```python
from build123d import *

# Parameters (mm, degrees)
PAD033_DEPTH            = 144
SKETCH060_R             = 1.5
POCKET025_DEPTH         = 7
POCKET026_DEPTH         = 4
SKETCH065_R             = 1.5
POCKET029_DEPTH         = 7
POCKET030_DEPTH         = 5
BODY018_ROLL_ANGLE      = 90
BODY018_PLACEMENT_ANGLE = 180


with BuildPart() as righthigh:
    # Sketch059 → Pad033 (new body)
    with BuildSketch(Plane.XZ):
        Polygon((0, 0), (0, 10), (-7, 10), (-7, 14), (4, 14), (4, 8), (7, 8), (7, -8), (4, -8), (4, -14), (-7, -14), (-7, -10), (0, -10), align=None)
    extrude(amount=PAD033_DEPTH)

    # Sketch060 (on Face6 of Pad033) → Pocket025 (cut)
    with BuildSketch(Plane(origin=(7, 0, 0), x_dir=(0, 0, 1), z_dir=(1, 0, 0))):
        with Locations((0, 120)):
            Circle(SKETCH060_R)
        with Locations((0, 20)):
            Circle(SKETCH060_R)
    extrude(amount=-POCKET025_DEPTH, mode=Mode.SUBTRACT)

    # Sketch061 (on Face12 of Pocket025) → Pocket026 (cut)
    with BuildSketch(Plane(origin=(7, 0, 0), x_dir=(0, 0, 1), z_dir=(1, 0, 0))):
        Polygon((3.176, 20), (1.588, 22.750497), (-1.588, 22.750497), (-3.176, 20), (-1.588, 17.249503), (1.588, 17.249503), align=None)
        Polygon((3.176, 120), (1.588, 122.750497), (-1.588, 122.750497), (-3.176, 120), (-1.588, 117.249503), (1.588, 117.249503), align=None)
    extrude(amount=-POCKET026_DEPTH, mode=Mode.SUBTRACT)

    # Sketch065 (on Face2 of Pocket026) → Pocket029 (cut)
    with BuildSketch(Plane(origin=(0, 0, 0), x_dir=(0, 0, -1), z_dir=(-1, 0, 0))):
        with Locations((0, 12.5)):
            Circle(SKETCH065_R)
        with Locations((0, 37.5)):
            Circle(SKETCH065_R)
        with Locations((0, 62.5)):
            Circle(SKETCH065_R)
        with Locations((0, 87.5)):
            Circle(SKETCH065_R)
        with Locations((0, 112.5)):
            Circle(SKETCH065_R)
        with Locations((0, 137.5)):
            Circle(SKETCH065_R)
    extrude(amount=-POCKET029_DEPTH, mode=Mode.SUBTRACT)

    # Sketch066 → Pocket030 (cut)
    with BuildSketch(Plane(origin=(0, 0, 0), x_dir=(0, 0, -1), z_dir=(-1, 0, 0))):
        Polygon((3.175366, 12.563434), (1.532748, 15.281665), (-1.642619, 15.218231), (-3.175366, 12.436566), (-1.532748, 9.718335), (1.642619, 9.781769), align=None)
        Polygon((3.175984, 37.50994), (1.579384, 40.255453), (-1.5966, 40.245513), (-3.175984, 37.49006), (-1.579384, 34.744547), (1.5966, 34.754487), align=None)
        Polygon((3.176, 62.500829), (1.587282, 65.250911), (-1.588718, 65.250082), (-3.176, 62.499171), (-1.587282, 59.749089), (1.588718, 59.749918), align=None)
        Polygon((3.176, 87.500019), (1.587984, 90.250506), (-1.588016, 90.250487), (-3.176, 87.499981), (-1.587984, 84.749494), (1.588016, 84.749513), align=None)
        Polygon((3.176, 112.5), (1.588, 115.250497), (-1.588, 115.250497), (-3.176, 112.5), (-1.588, 109.749503), (1.588, 109.749503), align=None)
        Polygon((3.176, 137.5), (1.588, 140.250497), (-1.588, 140.250497), (-3.176, 137.5), (-1.588, 134.749503), (1.588, 134.749503), align=None)
    extrude(amount=-POCKET030_DEPTH, mode=Mode.SUBTRACT)


with BuildPart() as righthigh_1:
    # Body018 roll: moved
    add(righthigh.part.rotate(Axis((0, 0, 0), (1, 0, 0)), BODY018_ROLL_ANGLE))


with BuildPart() as righthigh_2:
    # Body018 placement: moved
    add(righthigh_1.part.moved(Location((120, -275.5, 350))).rotate(Axis((120, -275.5, 350), (0, 0, 1)), BODY018_PLACEMENT_ANGLE))


with BuildPart() as lefthigh:
    # Part__Mirroring007: instance of RightHigh
    add(righthigh_2.part.mirror(Plane(origin=(0, 0, 0), x_dir=(0, -1, 0), z_dir=(1, 0, 0))))


solid = lefthigh.part
```
Model file for the job. Use its own axes, mm. A direction names the side the tool comes from. Coordinates: 2 decimals unless noted, no trailing zeros. Write each loop counter-clockwise with the first axis right and the second up, starting at its lowest first coordinate (ties: lowest second). Pieces come first, ordered by that corner, then holes. Notation, with made-up numbers: (-14, 47) - (0, 47) arc R12 ccw to (0, 52) - close; hole circle Ø5 at (78.25, 43). An arc over 180 degrees is marked (long way). One line per item, written item: value. Start each with the question number.
1. Slice it at A-A (z = 254.5). Write the cut outline in (x, y).
2. Flat gauge pins, fed straight in: pin 1 (6 mm diameter, centred on y = -274.5, z = 213, fed in from -X); pin 2 (1.7 mm diameter, centred on y = -274.5, z = 263.5, fed in from -X); pin 3 (6.5 mm diameter, centred on y = -287.5, z = 254, fed in from +X). Where does each tip first touch, or does it go through?
3. Mould opens along Y. For faces 4 (the flat face through (-116, -264, 279)), 5 (the flat face through (-114, -283.5, 279)), 6 (the flat face through (-117.535, -277.871, 213.895)) say: released by +Y, released by -Y, zero draft, split by the parting line, or undercut.
4. Probe line 1 (Y direction, x = -113.55, z = 262.5); line 2 (Y direction, x = -121.75, z = 233); line 3 (X direction, y = -287, z = 307.5). List the from-to ranges inside material, lowest first. Write a range as from..to.
5. Slice it at B-B (y = -282). Write the cut outline in (x, z), plus the area to 3 significant figures.
6. Tool access for faces 1 (the flat face through (-113, -275, 279)), 2 (the flat face through (-114.97, -277.89, 331.36)), 3 (the flat face through (-118, -275, 240.25)): list every direction of +Z, -Z, +X, -X, +Y, -Y with a clear straight run to the whole face (end or side of a thin tool).
7. Slice it at C-C (y = -275.5). Count the separate pieces of the cut face and the enclosed holes in it, plus the area to 3 significant figures.
Answers below:
1. outline: (-127, -289.5) - (-116, -289.5) - (-116, -283.5) - (-113, -283.5) - (-113, -267.5) - (-116, -267.5) - (-116, -261.5) - (-127, -261.5) - (-127, -265.5) - (-120, -265.5) - (-120, -285.5) - (-127, -285.5) - close
2. pin 1: stops at x = -120
2. pin 2: stops at x = -115
2. pin 3: stops at x = -116
3. face 4: zero draft
3. face 5: released by -Y
3. face 6: undercut
4. line 1: y = -283.5..-277, -274..-267.5
4. line 2: y = -289.5..-285.5, -265.5..-261.5
4. line 3: x = -127..-116
5. outline: (-120, 206) - (-113, 206) - (-113, 350) - (-120, 350) - close
5. area: 1,010 mm^2
6. face 1: +Z, -Z, +X, +Y, -Y
6. face 2: +X
6. face 3: -X
7. separate pieces: 9
7. enclosed holes: 0
7. area: 745 mm^2
